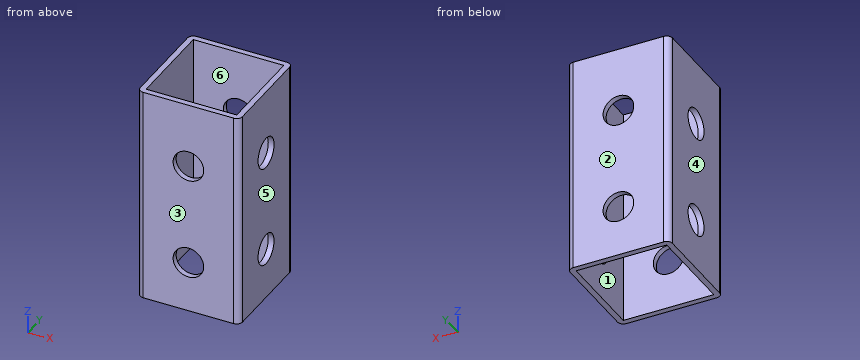
from build123d import *

# Parameters (mm, degrees)
SKETCH1_W                 = 42.2402
SKETCH1_H                 = 42.2402
BASE_EXTRUDE_DEPTH        = 101.6
HOLE1_START               = -23.8125
HOLE1_OUTLINE_R           = 7.14375
HOLE1_DEPTH               = 47.625
CIRPATTERN2_COUNT         = 2
CIRPATTERN2_ANGLE         = 90
LPATTERN1_COUNT           = 2
LPATTERN1_PITCH           = 47.625
LPATTERN1_START           = -23.8125
LPATTERN1_COPY_1_SKETCH_R = 7.14375
LPATTERN1_COPY_1_DEPTH    = 47.625


# Read off the part's stored shape, not the designer's step: Hole1
with BuildPart() as part:
    # Sketch1 → Base-Extrude (new body)
    with BuildSketch(Plane.XY):
        with BuildLine():
            Line((-23.8125, 21.1201), (-23.8125, -21.1201))
            ThreePointArc((-23.8125, -21.1201), (-23.023914298, -23.023914298), (-21.1201, -23.8125))
            Line((-21.1201, -23.8125), (21.1201, -23.8125))
            ThreePointArc((21.1201, -23.8125), (23.023914298, -23.023914298), (23.8125, -21.1201))
            Line((23.8125, -21.1201), (23.8125, 21.1201))
            ThreePointArc((23.8125, 21.1201), (23.023914298, 23.023914298), (21.1201, 23.8125))
            Line((21.1201, 23.8125), (-21.1201, 23.8125))
            ThreePointArc((-21.1201, 23.8125), (-23.023914298, 23.023914298), (-23.8125, 21.1201))
        make_face()
        Rectangle(SKETCH1_W, SKETCH1_H, mode=Mode.SUBTRACT)
    extrude(amount=BASE_EXTRUDE_DEPTH)

    # Hole1 outline → Hole1 (cut)
    with BuildSketch(Plane(origin=(0, 0, 0), x_dir=(1, 0, 0), z_dir=(0, 1, 0)).offset(HOLE1_START)):
        with Locations((0, -23.8125)):
            Circle(HOLE1_OUTLINE_R)
    hole1 = extrude(amount=HOLE1_DEPTH, mode=Mode.SUBTRACT)

    # CirPattern2: Hole1 ×2 about axis
    cirpattern2_axis = Axis((0, 0, -50), (0, 0, 1))
    for i in range(1, CIRPATTERN2_COUNT):
        add(hole1.rotate(cirpattern2_axis, i * CIRPATTERN2_ANGLE / (CIRPATTERN2_COUNT - 1)), mode=Mode.SUBTRACT)

    # LPattern1: Hole1 ×2
    with Locations(*[(0, 0, i * LPATTERN1_PITCH) for i in range(1, LPATTERN1_COUNT)]):
        add(hole1, mode=Mode.SUBTRACT)

    # LPattern1 copy 1 sketch → LPattern1 copy 1 (cut)
    with BuildSketch(Plane(origin=(0, 0, 47.625), x_dir=(0, 1, 0), z_dir=(-1, 0, 0)).offset(LPATTERN1_START)):
        with Locations((0, -23.8125)):
            Circle(LPATTERN1_COPY_1_SKETCH_R)
    extrude(amount=LPATTERN1_COPY_1_DEPTH, mode=Mode.SUBTRACT)


solid = part.part
Model file for the job. Use its own axes, mm. Face numbers are marked on the shaded views. A direction names the side the tool comes from. Round coordinates to 2 decimals unless told otherwise and drop trailing zeros. Order: outer loops, then holes, each group sorted by start corner. A loop starts at its lowest first (then second) coordinate and runs counter-clockwise, first axis right, second up. Notation, with made-up numbers: M -27,56.25 L 6,56.25 A4 cw 6,62.25 Z; hole C 52,21 d2. An arc over 180 degrees is marked long. Write each question's results on one line, items separated by ' | '. Start each with the question number.
(1) Which spindle directions (+Z, -Z, +X, -X, +Y, -Y) get a long thin tool onto all of the face, cutting with end or side? Do the marked faces 5 and 6. Say none if no direction does.
(2) Saw through at B-B, the plane x = 0. Give the cut face in (y, z), then the cut area to 3 significant figures.
(3) Probe probe 1 along Z at (x, y) = (-21.7, 0); probe 2 along Y at (x, z) = (-5, 64). List the from-to ranges inside material, lowest first. Write a range as from..to.
(4) Saw through at A-A, the plane y = 17.5. Give the cut face in (x, z), then the cut area to 3 significant figures.
(5) Drop flat-ended pins along their axis: pin 1 (11.5 mm diameter, centred on x = 0, z = 71.44, fed in from -Y); pin 2 (16.5 mm diameter, centred on x = 0, z = 23.81, fed in from -Y). Give the stop position or say it passes through.
(6) Saw through at C-C, the plane z = 28.5. Give the cut face in (x, y).
(7) Two-plate mould, pull along Y, no slides. Class the marked faces 1, 2, 3 and 4: pulls with the +Y half, pulls with the -Y half, needs draft (parallel to the pull), parting line crosses it, or undercut.
Established:
1) face 5: +Z, -Z, +X, +Y, -Y | face 6: +Z, -Z
2) outline: M -23.81,0 L -21.12,0 L -21.12,16.67 L -23.81,16.67 Z; M -23.81,30.96 L -21.12,30.96 L -21.12,64.29 L -23.81,64.29 Z; M -23.81,78.58 L -21.12,78.58 L -21.12,101.6 L -23.81,101.6 Z; M 21.12,0 L 23.81,0 L 23.81,16.67 L 21.12,16.67 Z; M 21.12,30.96 L 23.81,30.96 L 23.81,64.29 L 21.12,64.29 Z; M 21.12,78.58 L 23.81,78.58 L 23.81,101.6 L 21.12,101.6 Z | area: 393 mm^2
3) probe 1: z = 0..16.67, 30.96..64.29, 78.58..101.6 | probe 2: y = -23.81..-21.12, 21.12..23.81
4) outline: M -23.81,0 L -21.12,0 L -21.12,101.6 L -23.81,101.6 Z; M 21.12,0 L 23.81,0 L 23.81,101.6 L 21.12,101.6 Z | area: 547 mm^2
5) pin 1: passes through | pin 2: stops at y = -23.81
6) outline: M -23.81,-21.12 A2.69 ccw -21.12,-23.81 L -5.39,-23.81 L -5.39,-21.12 L -21.12,-21.12 L -21.12,-5.39 L -23.81,-5.39 Z; M -23.81,5.39 L -21.12,5.39 L -21.12,21.12 L -5.39,21.12 L -5.39,23.81 L -21.12,23.81 A2.69 ccw -23.81,21.12 Z; M 5.39,-23.81 L 21.12,-23.81 A2.69 ccw 23.81,-21.12 L 23.81,-5.39 L 21.12,-5.39 L 21.12,-21.12 L 5.39,-21.12 Z; M 5.39,21.12 L 21.12,21.12 L 21.12,5.39 L 23.81,5.39 L 23.81,21.12 A2.69 ccw 21.12,23.81 L 5.39,23.81 Z
7) face 1: undercut | face 2: pulls with the +Y half | face 3: pulls with the -Y half | face 4: needs draft
